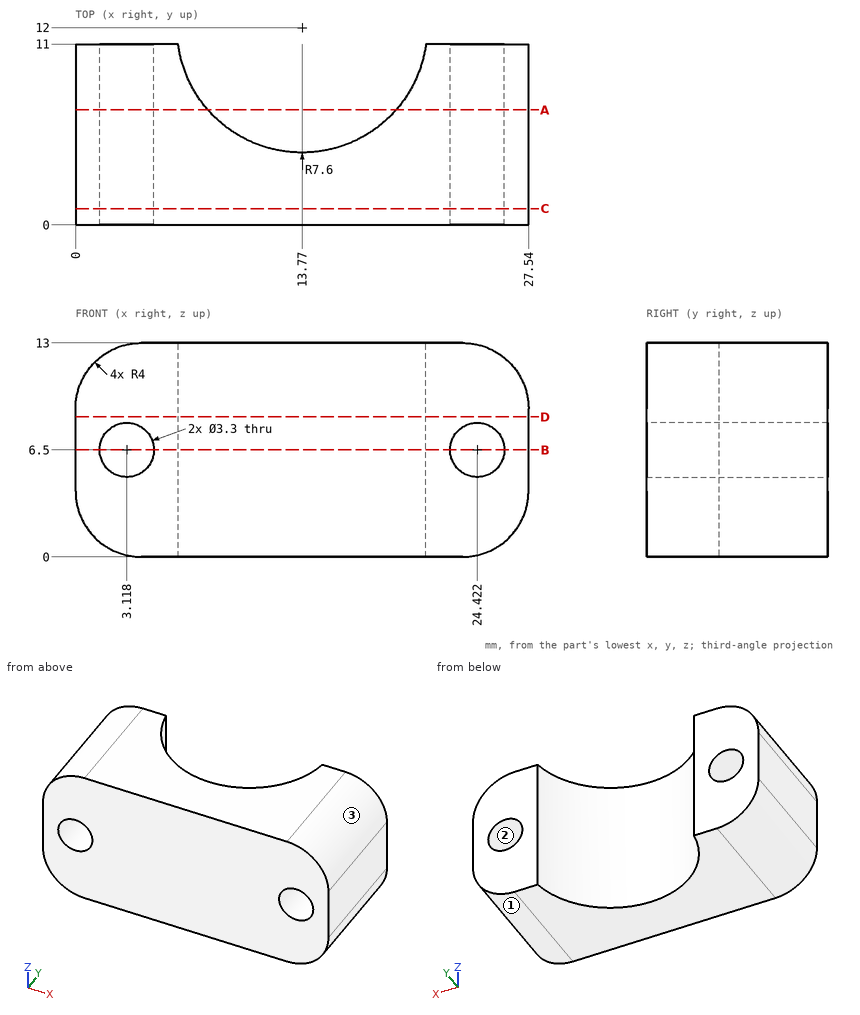
Design review of the part shown in the three views and the two pictorial views. Dimensions are in mm from the part's minimum x, y and z. Round coordinates to 2 decimals unless told otherwise and drop trailing zeros. Write each loop counter-clockwise with the first axis right and the second up, starting at its lowest first coordinate (ties: lowest second). Pieces come first, ordered by that corner, then holes. Notation, with made-up numbers: (-15, -13) -> (5, -13) arc R17 ccw to (5, -7) -> close; hole circle Ø7 at (20.5, 83). An arc over 180 degrees is marked (long way). One line per question, with ' | ' between items. Start each with the question number.
1) Wall thickness on line 1 along X through (y, z) = (2.5, 6.5); line 2 along X through (y, z) = (2.5, 5.75); line 3 along Z through (x, y) = (25, 2): over which ranges is each line inside the solid? List them lowest first.
2) Mouldability with a two-part tool opening along Z and no side actions: class the marked faces 1, 2 and 3 as +Z half, -Z half, draft (parallel to the pull), parting line (faces both ways), or undercut.
3) Add section A-A (y = 7). Write out the cut boundary in (x, z), and give its area (3 significant figures).
4) Add section B-B (z = 6.5). Write out the cut boundary in (x, y), and give its area (3 significant figures).
5) Add section D-D (z = 8.5). Write out the cut boundary in (x, y), and give its area (3 significant figures).
6) Add section C-C (y = 1). Write out the cut boundary in (x, z), and give its area (3 significant figures).
Reported:
1) line 1: x = 0 to 1.47, 4.77 to 22.77, 26.07 to 27.54 | line 2: x = 0 to 1.65, 4.59 to 22.95, 25.89 to 27.54 | line 3: z = 0.28 to 4.95, 8.05 to 12.72
2) face 1: -Z half | face 2: undercut | face 3: +Z half
3) outline: (0, 4) arc R4 ccw to (4, 0) -> (8.05, 0) -> (8.05, 13) -> (4, 13) arc R4 ccw to (0, 9) -> close; (19.49, 0) -> (23.54, 0) arc R4 ccw to (27.54, 4) -> (27.54, 9) arc R4 ccw to (23.54, 13) -> (19.49, 13) -> close; hole circle Ø3.3 at (3.12, 6.5); hole circle Ø3.3 at (24.42, 6.5) | area: 178 mm²
4) outline: (0, 0) -> (1.47, 0) -> (1.47, 11) -> (0, 11) -> close; (4.77, 0) -> (22.77, 0) -> (22.77, 11) -> (21.3, 11) arc R7.6 cw to (6.24, 11) -> (4.77, 11) -> close; (26.07, 0) -> (27.54, 0) -> (27.54, 11) -> (26.07, 11) -> close | area: 155 mm²
5) outline: (0, 0) -> (27.54, 0) -> (27.54, 11) -> (21.3, 11) arc R7.6 cw to (6.24, 11) -> (0, 11) -> close | area: 227 mm²
6) outline: (0, 4) arc R4 ccw to (4, 0) -> (23.54, 0) arc R4 ccw to (27.54, 4) -> (27.54, 9) arc R4 ccw to (23.54, 13) -> (4, 13) arc R4 ccw to (0, 9) -> close; hole circle Ø3.3 at (3.12, 6.5); hole circle Ø3.3 at (24.42, 6.5) | area: 327 mm²
